Can you work these out from the model? Positions are in its coordinate system, mm. A direction names the side the tool comes from. Coordinates: 2 decimals unless noted, no trailing zeros. Order: outer loops, then holes, each group sorted by start corner. A loop starts at its lowest first (then second) coordinate and runs counter-clockwise, first axis right, second up. Notation, with made-up numbers: (43.25, -36) -> (100.25, -36) arc R21 ccw to (100.25, -29) -> close; hole circle Ø11 at (42.5, 78). An arc over 180 degrees is marked (long way). Write item = value, one per line. Start each with the question number.
from build123d import *

# Parameters (mm, degrees)
BOSS_EXTRUDE1_DEPTH        = 10
FILLET1_R                  = 3
FILLET2_R                  = 6
SKETCH3_R                  = 2.5
CUT_EXTRUDE1_DEPTH         = 41.154825364
F_5_5_5_5_DIAMETER_HOLE1_D = 5.5


with BuildPart() as part:
    # Sketch1 → Boss-Extrude1 (new, symmetric)
    with BuildSketch(Plane.XY):
        Polygon((0, -17), (0, 17), (19.1, 17), (19.1, 32), (22.1, 32), (22.1, 14), (3, 14), (3, -14), (22.1, -14), (22.1, -32), (19.1, -32), (19.1, -17), align=None)
    extrude(amount=BOSS_EXTRUDE1_DEPTH, both=True)

    # Fillet1
    fillet1_edges = [part.edges().sort_by_distance(p)[0] for p in [
        (3, -14, 0),
        (19.1, -17, 0),
        (19.1, 17, 0),
        (3, 14, 0),
    ]]
    fillet(fillet1_edges, radius=FILLET1_R)

    # Fillet2
    fillet2_edges = [part.edges().sort_by_distance(p)[0] for p in [
        (22.1, -14, 0),
        (0, -17, 0),
        (0, 17, 0),
        (22.1, 14, 0),
    ]]
    fillet(fillet2_edges, radius=FILLET2_R)

    # Sketch3 → Cut-Extrude1 (cut, through all)
    with BuildSketch(Plane.ZY):
        Circle(SKETCH3_R)
    extrude(amount=-CUT_EXTRUDE1_DEPTH, mode=Mode.SUBTRACT)

    # Ø5.5 (5.5) Diameter Hole1 (through all)
    with Locations(Plane.ZY):
        with Locations((0, 26), (0, -26)):
            Hole(F_5_5_5_5_DIAMETER_HOLE1_D / 2)


solid = part.part
(1) Imagine slicing it at D-D (z = -6.75). Write out the boundary of the cut face in (x, y), plus the area to 3 significant figures.
(2) Thinking about a two-plate mould opening in Z: for faces 1 (the face through (2, 0, -10)), 2 (the face through (22.1, 29, 0)), 3 (the face through (2, 0, 10)), 4 (the face through (20.621, 28.727, 0.358)), which applies, +Z half, -Z half, draft (parallel to the pull), parting line (faces both ways), or undercut?
(3) For faces 5 (the face through (11, 17, 0)), 6 (the face through (3, 3, 0)), 7 (the face through (11, -17, 0)), which set-ups out of +Z, -Z, +X, -X, +Y, -Y let a thin tool reach every point of the face, with its end or its side?
(4) For P1, Ø3, axis at x = 10, z = -0.5, coming from the -Y side; P2, Ø3, axis at y = 0, z = 0, coming from the +X side (3 decimals); P3, Ø4, axis at y = 25.5, z = 2.5, coming from the -X side; P4, Ø10, axis at y = 1, z = -2, coming from the +X side, each with a flat end and sliding along its axis, tell me the tip position at first contact or that it passes through.
(5) Imagine slicing it at B-B (z = 0). Count the separate pieces of the cut face and the enclosed holes in it, plus the area to 3 significant figures.
(6) Imagine slicing it at A-A (y = 0). Write out the boundary of the cut face in (x, z), plus the area to 3 significant figures.
(7) If I drill on L1, parallel to Y at x = 14.25, z = 3; L2, parallel to Y at x = 21.25, z = -0.5; L3, parallel to X at y = -20, z = 8.25, over which ranges is the centre line in solid material (lowest first)? Write a range as from..to.
(8) Imagine slicing it at C-C (x = 12). Write out the boundary of the cut face in (y, z), plus the area to 3 significant figures.
Result set:
q1.outline = (0, -11) arc R6 ccw to (6, -17) -> (16.1, -17) arc R3 cw to (19.1, -20) -> (19.1, -32) -> (22.1, -32) -> (22.1, -20) arc R6 ccw to (16.1, -14) -> (6, -14) arc R3 cw to (3, -11) -> (3, 11) arc R3 cw to (6, 14) -> (16.1, 14) arc R6 ccw to (22.1, 20) -> (22.1, 32) -> (19.1, 32) -> (19.1, 20) arc R3 cw to (16.1, 17) -> (6, 17) arc R6 ccw to (0, 11) -> close
q1.area = 283 mm2
q2.face_1 = -Z half
q2.face_2 = draft
q2.face_3 = +Z half
q2.face_4 = undercut
q3.face_5 = +Z, -Z, -X, +Y
q3.face_6 = +Z, -Z, +X
q3.face_7 = +Z, -Z, -X, -Y
q4.P1 = -17
q4.P2 = through
q4.P3 = 19.1
q4.P4 = 3
q5.separate_pieces = 4
q5.enclosed_holes = 0
q5.area = 235 mm2
q6.outline = (0, -10) -> (3, -10) -> (3, -2.5) -> (0, -2.5) -> close; (0, 2.5) -> (3, 2.5) -> (3, 10) -> (0, 10) -> close
q6.area = 45.0 mm2
q7.L1 = -17..-14, 14..17
q7.L2 = -32..-28.7, -23.3..-16.92, 16.92..23.3, 28.7..32
q7.L3 = 19.1..22.1
q8.outline = (-17, -10) -> (-14, -10) -> (-14, 10) -> (-17, 10) -> close; (14, -10) -> (17, -10) -> (17, 10) -> (14, 10) -> close
q8.area = 120 mm2
